CAD build for the part. Positions are in the model's coordinates, mm. A direction names the side the tool comes from. Round coordinates to 2 decimals unless told otherwise and drop trailing zeros. Loops run counter-clockwise (first coordinate to the right, second up) from the corner with the lowest first, then second, coordinate; pieces in that order, holes last. Notation, with made-up numbers: (11.25, -31.75) - (29.25, -31.75) arc R22 ccw to (29.25, -8.75) - close; hole circle Ø2 at (-24, -12.75). An arc over 180 degrees is marked (long way). Use one line per item in the form item = value.
from build123d import *

# Parameters (mm, degrees)
SKETCH1_R           = 1.5
BOSS_EXTRUDE1_DEPTH = 3
FILLET1_R           = 1


with BuildPart() as part:
    # Sketch1 → Boss-Extrude1 (new body)
    with BuildSketch(Plane.XY):
        with BuildLine():
            Line((20.05, 5), (0, 5))
            ThreePointArc((0, 5), (-5, 0), (0, -5))
            Line((0, -5), (22, -5))
            Line((22, -5), (26.644435765, 1.851814361))
            ThreePointArc((26.644435765, 1.851814361), (24.805434743, 4.138784351), (22, 5))
            Line((22, 5), (20.05, 5))
        make_face()
        Circle(SKETCH1_R, mode=Mode.SUBTRACT)
        with Locations((22, 0)):
            Circle(SKETCH1_R, mode=Mode.SUBTRACT)
        with BuildLine():
            Line((46.409029503, 15.837507263), (20.05, 5))
            Line((20.05, 5), (22, 5))
            ThreePointArc((22, 5), (24.805434743, 4.138784351), (26.644435765, 1.851814361))
            Line((26.644435765, 1.851814361), (39.871788822, 7.125781662))
            Line((39.871788822, 7.125781662), (46.188488025, 4.540007042))
            Line((46.188488025, 4.540007042), (47.352932204, 4.337597171))
            Line((47.352932204, 4.337597171), (48.038244482, 5.300533868))
            Line((48.038244482, 5.300533868), (49.20268866, 5.098123997))
            Line((49.20268866, 5.098123997), (49.888000938, 6.061060693))
            Line((49.888000938, 6.061060693), (51.052445116, 5.858650822))
            Line((51.052445116, 5.858650822), (51.737757394, 6.821587519))
            Line((51.737757394, 6.821587519), (52.902201573, 6.619177648))
            Line((52.902201573, 6.619177648), (53.587513851, 7.582114344))
            Line((53.587513851, 7.582114344), (54.751958029, 7.379704473))
            Line((54.751958029, 7.379704473), (55.437270307, 8.34264117))
            Line((55.437270307, 8.34264117), (53.72608495, 12.504593197))
            Line((53.72608495, 12.504593197), (46.409029503, 15.837507263))
        make_face()
    extrude(amount=BOSS_EXTRUDE1_DEPTH)

    # Fillet1
    fillet1_edges = [part.edges().sort_by_distance(p)[0] for p in [
        (22, -5, 1.5),
        (20.05, 5, 1.5),
        (46.409029503, 15.837507263, 1.5),
        (53.72608495, 12.504593197, 1.5),
        (55.437270307, 8.34264117, 1.5),
        (46.188488025, 4.540007042, 1.5),
        (39.871788822, 7.125781662, 1.5),
        (26.644435765, 1.851814361, 1.5),
    ]]
    fillet(fillet1_edges, radius=FILLET1_R)


solid = part.part
1) Slice it at B-B (y = 0). Write the cut outline in (x, z).
Report:
outline = (-5, 0) - (-1.5, 0) - (-1.5, 3) - (-5, 3) - close; (1.5, 0) - (20.5, 0) - (20.5, 3) - (1.5, 3) - close; (23.5, 0) - (25.39, 0) - (25.39, 3) - (23.5, 3) - close
2) Tool access for faces 1 (the flat face through (53.24, 7.094, 1.479)), 2 (the cylindrical face through (-1.5, 0.07, 1.48)): list every direction of +Z, -Z, +X, -X, +Y, -Y with a clear straight run to the whole face (end or side of a thin tool).
Report:
face_1 = +Z, -Z, -Y
face_2 = +Z, -Z
3) Flat gauge pins, fed straight in: pin 1 (0.9 mm diameter, centred on x = 11, z = 1.5, fed in from +Y); pin 2 (1.5 mm diameter, centred on y = 13.5, z = 0.5, fed in from +X). Where does each tip first touch, or does it go through?
Report:
pin_1 = 5
pin_2 = 53.19
4) Slice it at C-C (x = 18). Write the cut outline in (y, z).
Report:
outline = (-5, 0) - (5, 0) - (5, 3) - (-5, 3) - close
5) Two-plate mould, pull along X, no slides. Class faces 3 (the flat face through (10, 5, 1)), 4 (the flat face through (54.162, 7.482, 1.479)), 5 (the flat face through (50.131, 14.142, 1.479)), 6 (the cylindrical face through (-5, 0, 1)): +X half, -X half, draft (parallel to the pull), parting line (faces both ways), or undercut.
Report:
face_3 = draft
face_4 = undercut
face_5 = +X half
face_6 = -X half
6) Slice it at D-D (y = -3.25). Write the cut outline in (x, z), plus the area to 3 significant figures.
Report:
outline = (-3.8, 0) - (23.19, 0) - (23.19, 3) - (-3.8, 3) - close
area = 81.0 mm^2
7) Drill centre lines: probe 1 along Y at (x, z) = (0, 2.25); probe 2 along X at (y, z) = (0.5, 0.75); probe 3 along Y at (x, z) = (7, 0.4). Where is each one in solid material? Low to high.
Report:
probe_1 = -5 to -1.5, 1.5 to 5
probe_2 = -4.97 to -1.41, 1.41 to 20.59, 23.41 to 25.73
probe_3 = -5 to 5
8) Slice it at A-A (z = 1.55). State how many separate pieces and enclosed holes the cut face has, plus the area to 3 significant figures.
Report:
separate_pieces = 1
enclosed_holes = 2
area = 486 mm^2
